Verification items for the finished model (mm, model axes). A direction names the side the tool comes from. Coordinates: 2 decimals unless noted, no trailing zeros. Order: outer loops, then holes, each group sorted by start corner. A loop starts at its lowest first (then second) coordinate and runs counter-clockwise, first axis right, second up. Notation, with made-up numbers: (85.5, 59) - (94.5, 59) arc R9 ccw to (94.5, 76) - close; hole circle Ø2 at (-2.5, -33.75). An arc over 180 degrees is marked (long way). Answer as CSV lines item,"result". Start each with the question number.
1. Section check D-D (y = -17). Record the cut outline in (x, z), and give its area (3 significant figures).
2. Material ranges on L1, parallel to Z at x = 1, y = 8.5; L2, parallel to X at y = -13.5, z = 0.25; L3, parallel to X at y = -21.5, z = -3.75, recorded low to high. Write a range as [from, to].
3. Set-up check for faces 5 (the flat face through (0, 31, -13)), 6 (the flat face through (3.75, -34, -6)), 7 (the flat face through (-8, -31.25, -6)): record each of +Z, -Z, +X, -X, +Y, -Y from which the full face is reachable in a straight line by a thin tool's end or side.
4. Section check A-A (y = -35). Record the cut outline in (x, z).
5. Section check B-B (z = -2). Record the cut outline in (x, y), and give its area (3 significant figures).
6. Go/stop test with flat-tipped pins: pin 1 (4 mm diameter, centred on y = 33.5, z = -8.5, fed in from -X); pin 2 (3 mm diameter, centred on y = 3, z = -11.5, fed in from +X); pin 3 (6 mm diameter, centred on x = 7, z = -8, fed in from -Y). Record where each tip stops, or that it passes through.
7. Section check C-C (x = -40.5). Record the cut outline in (y, z), and give its area (3 significant figures).
8. Mould release check, pull along Z, two halves, no side actions. Record for faces 1 (the flat face through (-3.75, 34, -6)), 2 (the flat face through (-8, 31.25, -6)), 3 (the flat face through (-28, 31, -14)), 4 (the cylindrical face through (-0.08, 39.75, -5.92)): pulls with the +Z half, pulls with the -Z half, needs draft (parallel to the pull), parting line crosses it, or undercut.
from build123d import *

# Parameters (mm, degrees)
SKETCH_1_W          = 28
SKETCH_1_H          = 85.5
EXTRUDE_1_DEPTH     = 2
SKETCH_2_W          = 15
SKETCH_2_H          = 45
SKETCH_2_W_2        = 10
SKETCH_2_H_2        = 7
CUT_EXTRUDE_1_DEPTH = 1
SKETCH_3_W          = 7.5
SKETCH_3_H          = 62.5
SKETCH_3_W_2        = 7.75
EXTRUDE_2_DEPTH     = 12
EXTRUDE_3_DEPTH     = 2


with BuildPart() as part:
    # 草图1 → 凸台-拉伸1 (new body)
    with BuildSketch(Plane.XY):
        Rectangle(SKETCH_1_W, SKETCH_1_H)
    extrude(amount=EXTRUDE_1_DEPTH)

    # 草图2 → 切除-拉伸1 (cut)
    with BuildSketch(Plane.XY.offset(2)):
        with Locations((0, 9.75)):
            Rectangle(SKETCH_2_W, SKETCH_2_H)
        with Locations((0, -4.25)):
            Rectangle(SKETCH_2_W_2, SKETCH_2_H_2, mode=Mode.SUBTRACT)
    extrude(amount=-CUT_EXTRUDE_1_DEPTH, mode=Mode.SUBTRACT)

    # 草图3 → 凸台-拉伸2 (add)
    with BuildSketch(Plane(origin=(0, 0, 0), x_dir=(-1, 0, 0), z_dir=(0, 0, -1))):
        Rectangle(SKETCH_3_W, SKETCH_3_H)
        with Locations((-7.625, 0)):
            Rectangle(SKETCH_3_W_2, SKETCH_3_H)
        with Locations((7.625, 0)):
            Rectangle(SKETCH_3_W_2, SKETCH_3_H)
        with BuildLine():
            Line((-3.75, 36), (-3.75, 31.25))
            Line((-3.75, 31.25), (3.75, 31.25))
            Line((3.75, 31.25), (3.75, 36))
            ThreePointArc((3.75, 36), (0, 39.75), (-3.75, 36))
        make_face()
        with BuildLine():
            Line((3.75, -31.25), (-3.75, -31.25))
            Line((-3.75, -31.25), (-3.75, -36))
            ThreePointArc((-3.75, -36), (0, -39.75), (3.75, -36))
            Line((3.75, -36), (3.75, -31.25))
        make_face()
    extrude(amount=EXTRUDE_2_DEPTH)

    # 草图4 → 凸台-拉伸3 (add)
    with BuildSketch(Plane(origin=(0, 0, -12), x_dir=(-1, 0, 0), z_dir=(0, 0, -1))):
        with BuildLine():
            Line((0, 36), (53, 36))
            ThreePointArc((53, 36), (55.121320344, 35.121320344), (56, 33))
            Line((56, 33), (56, 29))
            ThreePointArc((56, 29), (55.121320344, 26.878679656), (53, 26))
            Line((53, 26), (0, 26))
            Line((0, 26), (0, 36))
        make_face()
    extrude(amount=EXTRUDE_3_DEPTH)


solid = part.part
Evaluation:
1,outline,"(-14, 0) - (-11.5, 0) - (-11.5, -12) - (11.5, -12) - (11.5, 0) - (14, 0) - (14, 2) - (-14, 2) - close"
1,area,"332 mm²"
2,L1,"z = [-12, 1]"
2,L2,"x = [-14, 14]"
2,L3,"x = [-11.5, 11.5]"
3,face 5,"-Z, +X, +Y, -Y"
3,face 6,"-Z, +X, -Y"
3,face 7,"-Z, -X, -Y"
4,outline,"(-14, 0) - (-3.75, 0) - (-3.75, -12) - (3.75, -12) - (3.75, 0) - (14, 0) - (14, 2) - (-14, 2) - close"
5,outline,"(-11.5, -31.25) - (-3.75, -31.25) - (-3.75, -36) arc R3.75 ccw to (3.75, -36) - (3.75, -31.25) - (11.5, -31.25) - (11.5, 31.25) - (3.75, 31.25) - (3.75, 36) arc R3.75 ccw to (-3.75, 36) - (-3.75, 31.25) - (-11.5, 31.25) - close"
5,area,"1,550 mm²"
6,pin 1,"stops at x = -3.75"
6,pin 2,"stops at x = 11.5"
6,pin 3,"stops at y = -31.25"
7,outline,"(26, -14) - (36, -14) - (36, -12) - (26, -12) - close"
7,area,"20.0 mm²"
8,face 1,"undercut"
8,face 2,"undercut"
8,face 3,"pulls with the -Z half"
8,face 4,"needs draft"
